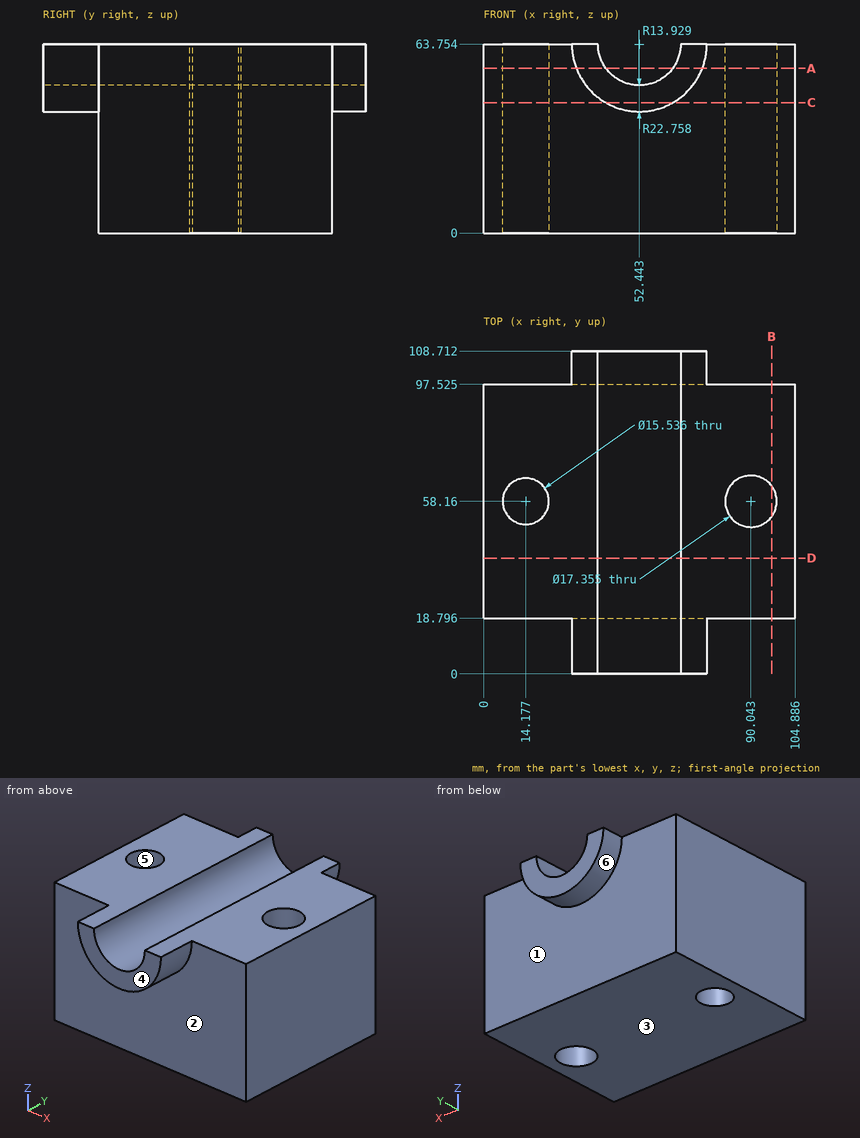
Geometry check sheet. Reference: drawing and pictorial views, mm from the part's lowest x, y, z. A direction names the side the tool comes from. Give positions to 0.01 mm unless a question says otherwise; leave off trailing zeros. Write each loop counter-clockwise with the first axis right and the second up, starting at its lowest first coordinate (ties: lowest second). Pieces come first, ordered by that corner, then holes.
Item 1: Cross-section at A-A (z = 55.5). Enter the section's corners in (x, y) (1 decimal), and give its area (3 significant figures).
Item 2: Draft check along Y on the marked faces 4, 5 and 6. Enter one of: released by +Y, released by -Y, zero draft, split by the parting line, or undercut.
Item 3: Cross-section at D-D (y = 39). Enter the section's corners in (x, z) (1 decimal), and give its area (3 significant figures).
Item 4: Access from +Z, -Z, +X, -X, +Y, -Y to the whole of each face (thin tool, end or side, straight path). Record for the marked faces 1, 2 and 3.
Item 5: Scan lines: L1, parallel to X at y = 57, z = 14 (1 decimal); L2, parallel to Y at x = 64, z = 18.5 (1 decimal); L3, parallel to X at y = 52, z = 36.5 (1 decimal). Record each from-to range of solid material in increasing order.
Item 6: Cross-section at C-C (z = 44). Enter the section's corners in (x, y) (1 decimal), and give its area (3 significant figures).
Item 7: Gauge pin test, flat ends, axial feed: pin 1 (19 mm diameter, centred on x = 39, z = 32, fed in from -Y); pin 2 (2 mm diameter, centred on x = 48.5, z = 33, fed in from +Y) (1 decimal); pin 3 (20 mm diameter, centred on x = 90.04, y = 58.16, fed in from +Z). Record the tip position at first contact, or that the pin passes through.
Item 8: Cross-section at B-B (x = 97). Enter the section's corners in (y, z) (1 decimal).
Report:
1. outline: (0, 18.8) - (31.2, 18.8) - (31.2, 0) - (41.2, 0) - (41.2, 108.7) - (31.2, 108.7) - (31.2, 97.5) - (0, 97.5) - close; (63.7, 0) - (73.7, 0) - (73.7, 18.8) - (104.9, 18.8) - (104.9, 97.5) - (73.7, 97.5) - (73.7, 108.7) - (63.7, 108.7) - close; hole circle Ø15.5 at (14.2, 58.2); hole circle Ø17.4 at (90, 58.2)
1. area: 6,660 mm2
2. face 4: released by -Y
2. face 5: undercut
2. face 6: zero draft
3. outline: (0, 0) - (104.9, 0) - (104.9, 63.8) - (66.4, 63.8) arc R13.9 cw to (38.5, 63.8) - (0, 63.8) - close
3. area: 6,380 mm2
4. face 1: -Z, +Y
4. face 2: -Z, -Y
4. face 3: -Z, +X, -X, +Y, -Y
5. L1: x = 0 to 6.5, 21.9 to 81.4, 98.6 to 104.9
5. L2: y = 18.8 to 97.5
5. L3: x = 0 to 9.4, 18.9 to 83.9, 96.2 to 104.9
6. outline: (0, 18.8) - (41.1, 18.8) - (41.1, 0) - (63.7, 0) - (63.7, 18.8) - (104.9, 18.8) - (104.9, 97.5) - (63.7, 97.5) - (63.7, 108.7) - (41.1, 108.7) - (41.1, 97.5) - (0, 97.5) - close; hole circle Ø15.5 at (14.2, 58.2); hole circle Ø17.4 at (90, 58.2)
6. area: 8,510 mm2
7. pin 1: stops at y = 18.8
7. pin 2: stops at y = 97.5
7. pin 3: stops at z = 63.75
8. outline: (18.8, 0) - (53, 0) - (53, 63.8) - (18.8, 63.8) - close; (63.3, 0) - (97.5, 0) - (97.5, 63.8) - (63.3, 63.8) - close
